Build history of the part. All positions in model axes, mm. Round coordinates to 2 decimals unless told otherwise and drop trailing zeros. Write each loop counter-clockwise with the first axis right and the second up, starting at its lowest first coordinate (ties: lowest second). Pieces come first, ordered by that corner, then holes. Notation, with made-up numbers: M 46.5,8 L 88.5,8 A13 ccw 88.5,14 Z; hole C 10,-29.75 d11. An arc over 180 degrees is marked long. Use a Markdown table: item, result.
from build123d import *

# Parameters (mm, degrees)
SKETCH1_W           = 190
SKETCH1_H           = 45
BOSS_EXTRUDE1_DEPTH = 10
SKETCH2_R           = 4
CUT_EXTRUDE1_DEPTH  = 10
SKETCH3_W           = 30
SKETCH3_H           = 45
CUT_EXTRUDE2_DEPTH  = 10
FILLET1_R           = 18
FILLET2_R           = 22


with BuildPart() as part:
    # Sketch1 → Boss-Extrude1 (new body)
    with BuildSketch(Plane(origin=(0, 0, 0), x_dir=(1, 0, 0), z_dir=(0, 1, 0))):
        Rectangle(SKETCH1_W, SKETCH1_H)
    extrude(amount=BOSS_EXTRUDE1_DEPTH)

    # Sketch2 → Cut-Extrude1 (cut)
    with BuildSketch(Plane(origin=(0, 10, 0), x_dir=(1, 0, 0), z_dir=(0, 1, 0))):
        with Locations(Location((-43, 0, 0), (0, 0, 270))):
            Circle(SKETCH2_R)
        with Locations(Location((77, 0, 0), (0, 0, 270))):
            Circle(SKETCH2_R)
    extrude(amount=-CUT_EXTRUDE1_DEPTH, mode=Mode.SUBTRACT)

    # Sketch3 → Cut-Extrude2 (cut)
    with BuildSketch(Plane(origin=(0, 10, 0), x_dir=(1, 0, 0), z_dir=(0, 1, 0))):
        Polygon((95, -22.5), (-5, -22.5), (95, -17.5), align=None)
        Polygon((-5, 22.5), (95, 17.5), (95, 22.5), align=None)
        with Locations((-80, 0)):
            Rectangle(SKETCH3_W, SKETCH3_H)
    extrude(amount=-CUT_EXTRUDE2_DEPTH, mode=Mode.SUBTRACT)

    # Fillet1
    fillet1_edges = [part.edges().sort_by_distance(p)[0] for p in [
        (95, 5, -17.5),
        (95, 5, 17.5),
    ]]
    fillet(fillet1_edges, radius=FILLET1_R)

    # Fillet2
    fillet2_edges = [part.edges().sort_by_distance(p)[0] for p in [
        (-65, 5, -22.5),
        (-65, 5, 22.5),
    ]]
    fillet(fillet2_edges, radius=FILLET2_R)


solid = part.part
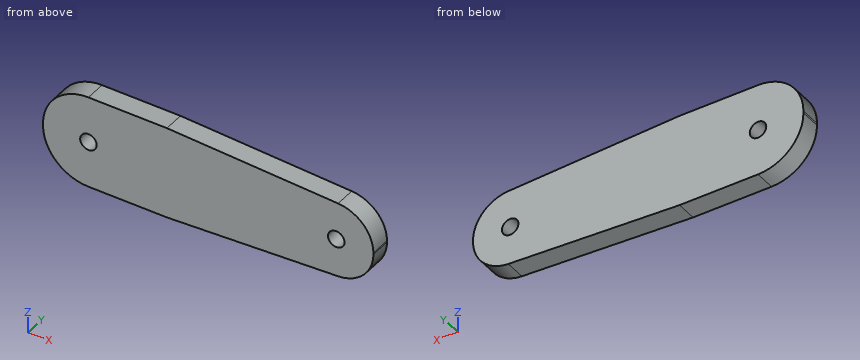
Q1. Cut at A-A on y = 6.5. Give the cut face in (x, z).
Response values:
| item | result |
|---|---|
| outline | M -65,-0.5 A22 ccw -43,-22.5 L -5,-22.5 L 77.9,-18.36 A18 ccw 95,-0.38 L 95,0.38 A18 ccw 77.9,18.36 L -5,22.5 L -43,22.5 A22 ccw -65,0.5 Z; hole C -43,0 d8; hole C 77,0 d8 |
Q2. Drill centre lines: L1, parallel to X at y = 7, z = 0; L2, parallel to Z at x = -45, y = 2; L3, parallel to X at y = 7.75, z = -3. Where is each one in solid material? Low to high.
Response values:
| item | result |
|---|---|
| L1 | x = -65 to -47, -39 to 73, 81 to 95 |
| L2 | z = -22.41 to -3.46, 3.46 to 22.41 |
| L3 | x = -64.86 to -45.65, -40.35 to 74.35, 79.65 to 94.81 |
Q3. Drop flat-ended pins along their axis: P1, Ø3, axis at y = 3.5, z = -8, coming from the +X side; P2, Ø4, axis at y = 8, z = -18, coming from the +X side; P3, Ø2, axis at x = 71, y = 2, coming from the -Z side. Give the stop position or say it passes through.
Response values:
| item | result |
|---|---|
| P1 | stops at x = 93.93 |
| P2 | stops at x = 85.94 |
| P3 | stops at z = -18.75 |
Q4. Cut at B-B on x = 46. Give the cut face in (y, z), and give its area (3 significant figures).
Response values:
| item | result |
|---|---|
| outline | M 0,-19.95 L 10,-19.95 L 10,19.95 L 0,19.95 Z |
| area | 399 mm2 |
Q5. Cut at C-C on z = 9.5. Give the cut face in (x, y).
Response values:
| item | result |
|---|---|
| outline | M -63.07,0 L 92.52,0 L 92.52,10 L -63.07,10 Z |
